from build123d import *

# Parameters (mm, degrees)
FILLET1_R               = 1
CHAMFER1_SIZE           = 1
FILLET2_R               = 5
SKETCH3_W               = 2
SKETCH3_H               = 12
CUT_EXTRUDE1_DEPTH      = 12
SKETCH4_R               = 2.55
CUT_EXTRUDE2_DEPTH      = 19
CUT_EXTRUDE2_DEPTH_BACK = 19


with BuildPart() as part:
    # Sketch1 → Revolve1 (revolve)
    with BuildSketch(Plane.XY):
        Polygon((18, 0), (5.25, 0), (5.25, 3), (10.25, 3), (10.25, 30), (18, 30), align=None)
    revolve(axis=Axis((0, -427.095192794, 0), (0, 1, 0)))

    # Fillet1
    fillet1_edges = [part.edges().sort_by_distance(p)[0] for p in [
        (-10.25, 3, 0),
    ]]
    fillet(fillet1_edges, radius=FILLET1_R)

    # Chamfer1
    chamfer1_edges = [part.edges().sort_by_distance(p)[0] for p in [
        (-18, 30, 0),
        (-10.25, 30, 0),
    ]]
    chamfer(chamfer1_edges, length=CHAMFER1_SIZE)

    # Fillet2
    fillet2_edges = [part.edges().sort_by_distance(p)[0] for p in [
        (-18, 0, 0),
    ]]
    fillet(fillet2_edges, radius=FILLET2_R)

    # Sketch3 → Cut-Extrude1 (cut)
    with BuildSketch(Plane(origin=(0, 30, 0), x_dir=(1, 0, 0), z_dir=(0, 1, 0))):
        with BuildLine():
            Line((-13.15, 4.05), (-9.415943925, 4.05))
            ThreePointArc((-9.415943925, 4.05), (-10.25, 0), (-9.415943925, -4.05))
            Line((-9.415943925, -4.05), (-13.15, -4.05))
            Line((-13.15, -4.05), (-13.15, 4.05))
        make_face()
        with BuildLine():
            Line((13.15, -4.05), (13.15, 4.05))
            Line((13.15, 4.05), (9.415943925, 4.05))
            ThreePointArc((9.415943925, 4.05), (10.25, 0), (9.415943925, -4.05))
            Line((9.415943925, -4.05), (13.15, -4.05))
        make_face()
        with Locations((17.970562748, 0)):
            Rectangle(SKETCH3_W, SKETCH3_H)
        with Locations((-17.970562748, 0)):
            Rectangle(SKETCH3_W, SKETCH3_H)
    extrude(amount=-CUT_EXTRUDE1_DEPTH, mode=Mode.SUBTRACT)

    # Sketch4 → Cut-Extrude2 (cut, two sides)
    with BuildSketch(Plane(origin=(0, 0, 0), x_dir=(0, 0, -1), z_dir=(1, 0, 0))) as cut_extrude2_sk:
        with Locations((0, 22.5)):
            Circle(SKETCH4_R)
    extrude(amount=CUT_EXTRUDE2_DEPTH, mode=Mode.SUBTRACT)
    extrude(cut_extrude2_sk.sketch, amount=-CUT_EXTRUDE2_DEPTH_BACK, mode=Mode.SUBTRACT)


solid = part.part
Check sheet for the modelled part. Datum: model origin and axes. Units: mm. A direction names the side the tool comes from. Round coordinates to 2 decimals unless told otherwise and drop trailing zeros. Loops run counter-clockwise (first coordinate to the right, second up) from the corner with the lowest first, then second, coordinate; pieces in that order, holes last. Notation, with made-up numbers: (78, 43) -> (117, 43) arc R11 cw to (117, 58) -> close; hole circle Ø1 at (-5, 83.25). An arc over 180 degrees is marked (long way). Put each result on its own line as item: value. Start each with the question number.
1. Section check C-C (y = 8.5). Enter the section's corners in (x, z), plus the area to 3 significant figures.
2. Access from +Z, -Z, +X, -X, +Y, -Y to the whole of each face (thin tool, end or side, straight path). Record for faces 4 (the face through (16.971, 25.4, 0.1)), 5 (the face through (-16.971, 25.4, 0.1)), 6 (the face through (-4, 3, 4)).
3. Section check B-B (x = 0). Enter the section's corners in (y, z).
4. Scan lines: probe 1 along Z at (x, y) = (0, 15.25); probe 2 along Y at (x, z) = (1.5, 6.5); probe 3 along X at (y, z) = (18.25, -2). Record each from-to range of solid material in increasing order.
5. Section check A-A (y = 22.5). Enter the section's corners in (x, z).
6. Draft check along Y on faces 1 (the face through (-13.15, 25.4, 0.1)), 2 (the face through (-0.18, 29.17, 10.42)), 3 (the face through (-15.03, 25.03, 0.33)). Enter one of: +Y half, -Y half, draft (parallel to the pull), parting line (faces both ways), or undercut.
7. Gauge pin test, flat ends, axial feed: pin 1 (4 mm diameter, centred on y = 20, z = 12.5, fed in from +X); pin 2 (6 mm diameter, centred on y = 22.5, z = 0, fed in from -X); pin 3 (13 mm diameter, centred on y = 25, z = -0.5, fed in from +X). Record the tip position at first contact, or that the pin passes through.
8. Section check D-D (z = -1.5). Give the number of separate pieces and of enclosed holes in the cut face, plus the area to 3 significant figures.
Findings:
1. outline: circle Ø36 at (0, 0); hole circle Ø20.5 at (0, 0)
1. area: 688 mm^2
2. face 4: +Z, -Z, +X, +Y
2. face 5: +Z, -Z, -X, +Y
2. face 6: +Y
3. outline: (0, -13) arc R5 ccw to (5, -18) -> (29, -18) -> (30, -17) -> (30, -11.25) -> (29, -10.25) -> (4, -10.25) arc R1 cw to (3, -9.25) -> (3, -5.25) -> (0, -5.25) -> close; (0, 5.25) -> (3, 5.25) -> (3, 9.25) arc R1 cw to (4, 10.25) -> (29, 10.25) -> (30, 11.25) -> (30, 17) -> (29, 18) -> (5, 18) arc R5 ccw to (0, 13) -> close
4. probe 1: z = -18 to -10.25, 10.25 to 18
4. probe 2: y = 0 to 3
4. probe 3: x = -16.97 to -13.15, 13.15 to 16.97
5. outline: (-16.97, -6) arc R18 ccw to (16.97, -6) -> (16.97, -2.55) -> (13.15, -2.55) -> (13.15, -4.05) -> (9.42, -4.05) arc R10.25 cw to (-9.42, -4.05) -> (-13.15, -4.05) -> (-13.15, -2.55) -> (-16.97, -2.55) -> close; (-16.97, 2.55) -> (-13.15, 2.55) -> (-13.15, 4.05) -> (-9.42, 4.05) arc R10.25 cw to (9.42, 4.05) -> (13.15, 4.05) -> (13.15, 2.55) -> (16.97, 2.55) -> (16.97, 6) arc R18 ccw to (-16.97, 6) -> close
6. face 1: draft
6. face 2: +Y half
6. face 3: undercut
7. pin 1: stops at x = 14.62
7. pin 2: stops at x = -16.97
7. pin 3: stops at x = 16.97
8. separate pieces: 4
8. enclosed holes: 0
8. area: 361 mm^2
